CAD build for the part. Positions are in the model's coordinates, mm. A direction names the side the tool comes from. Coordinates: 2 decimals unless noted, no trailing zeros. Order: outer loops, then holes, each group sorted by start corner. A loop starts at its lowest first (then second) coordinate and runs counter-clockwise, first axis right, second up. Notation, with made-up numbers: M 38.5,-13 L 81.5,-13 A29 ccw 81.5,22 Z; hole C 87.25,46 d7. An arc over 180 degrees is marked long. Write item = value, one per line.
from build123d import *
from build123d.topology import SkipClean

# Parameters (mm, degrees)
BOSS_EXTRUDE1_DEPTH = 5.1
SKETCH2_W           = 14.45
SKETCH2_H           = 1.1
CUT_EXTRUDE1_DEPTH  = 23.625704409
SKETCH3_W           = 0.825
SKETCH3_H           = 1.1
CUT_EXTRUDE2_DEPTH  = 10
FILLET1_R           = 0.1
SKETCH4_W           = 4.1
SKETCH4_H           = 5.1
CUT_EXTRUDE3_DEPTH  = 10


with BuildPart() as part:
    # Sketch1 → Boss-Extrude1 (new body)
    with BuildSketch(Plane(origin=(0, 0, 0), x_dir=(1, 0, 0), z_dir=(0, 1, 0))):
        with BuildLine():
            Line((20.1, 4.525), (0, 4.525))
            Line((0, 4.525), (0, 2.175))
            ThreePointArc((0, 2.175), (1.537957249, 1.537957249), (2.175, 0))
            Line((2.175, 0), (20.1, 0))
            Line((20.1, 0), (20.1, 4.525))
        make_face()
        with BuildLine():
            Line((20.1, 0), (2.175, 0))
            ThreePointArc((2.175, 0), (1.537957249, -1.537957249), (0, -2.175))
            Line((0, -2.175), (0, -4.525))
            Line((0, -4.525), (20.1, -4.525))
            Line((20.1, -4.525), (20.1, 0))
        make_face()
    extrude(amount=BOSS_EXTRUDE1_DEPTH)

    # Sketch2 → Cut-Extrude1 (cut, through all)
    with BuildSketch(Plane.XY.offset(4.525)):
        with Locations((0, 4.55)):
            Rectangle(SKETCH2_W, SKETCH2_H)
    extrude(amount=-CUT_EXTRUDE1_DEPTH, mode=Mode.SUBTRACT)

    # Sketch3 → Cut-Extrude2 (cut)
    with BuildSketch(Plane.XY.offset(4.525)):
        with Locations((8.769642857, 4.55)):
            Rectangle(SKETCH3_W, SKETCH3_H)
        with Locations((10.726785714, 4.55)):
            Rectangle(SKETCH3_W, SKETCH3_H)
        with Locations((12.683928571, 4.55)):
            Rectangle(SKETCH3_W, SKETCH3_H)
        with Locations((14.641071429, 4.55)):
            Rectangle(SKETCH3_W, SKETCH3_H)
        with Locations((16.598214286, 4.55)):
            Rectangle(SKETCH3_W, SKETCH3_H)
        with Locations((18.555357143, 4.55)):
            Rectangle(SKETCH3_W, SKETCH3_H)
    extrude(amount=-CUT_EXTRUDE2_DEPTH, mode=Mode.SUBTRACT)

    # Fillet1
    fillet1_edges = [part.edges().sort_by_distance(p)[0] for p in [
        (14.228571429, 4, 0),
        (15.053571429, 4, 0),
        (17.010714286, 5.1, 0),
        (16.185714286, 5.1, 0),
        (16.185714286, 4, 0),
        (17.010714286, 4, 0),
        (18.967857143, 5.1, 0),
        (18.142857143, 5.1, 0),
        (18.142857143, 4, 0),
        (18.967857143, 4, 0),
        (20.1, 5.1, 0),
        (7.225, 4, 0),
        (7.225, 5.1, 0),
        (9.182142857, 5.1, 0),
        (8.357142857, 5.1, 0),
        (8.357142857, 4, 0),
        (9.182142857, 4, 0),
        (11.139285714, 5.1, 0),
        (10.314285714, 5.1, 0),
        (10.314285714, 4, 0),
        (11.139285714, 4, 0),
        (13.096428571, 5.1, 0),
        (12.271428571, 5.1, 0),
        (12.271428571, 4, 0),
        (13.096428571, 4, 0),
        (15.053571429, 5.1, 0),
        (14.228571429, 5.1, 0),
    ]]
    fillet(fillet1_edges, radius=FILLET1_R)

    # Mirror3: part across plane


with BuildPart() as part_1:
    with SkipClean():  # the faces are left unmerged after this step: merging them gives an invalid solid
        add(part.part)
        add(part.part.mirror(Plane(origin=(0, 5.1, 0), x_dir=(0, 0, 1), z_dir=(1, 0, 0))))

    # Sketch4 → Cut-Extrude3 (cut)
    with SkipClean():  # the faces are left unmerged after this step: merging them gives an invalid solid
        with BuildSketch(Plane.XY.offset(4.525)):
            with Locations((18.05, 2.55)):
                Rectangle(SKETCH4_W, SKETCH4_H)
            with Locations((-18.05, 2.55)):
                Rectangle(SKETCH4_W, SKETCH4_H)
        extrude(amount=-CUT_EXTRUDE3_DEPTH, mode=Mode.SUBTRACT)


solid = part_1.part
(1) Pull direction X, two halves, no side cores. Call faces 3 (the face through (15.054, 4.5, 0.1)), 4 (the face through (10, 5.1, 0)), 5 (the face through (-16, 3, 0)): +X half, -X half, draft (parallel to the pull), parting line (faces both ways), or undercut.
Evaluation:
face_3 = undercut
face_4 = draft
face_5 = -X half
(2) Wall check: line 1 (Y direction, x = -5.5, z = 1.25); line 2 (X direction, y = 3.1, z = -1.75); line 3 (X direction, y = 1.45, z = 2). Give the ranges that are in metal, low to high. Write a range as from..to.
Evaluation:
line_1 = 0..4
line_2 = -16..-1.29, 1.29..16
line_3 = -16..-0.85, 0.85..16
(3) Tool access for faces 1 (the face through (12, 5.1, 0)), 2 (the face through (8.357, 4.5, 0.1)): list every direction of +Z, -Z, +X, -X, +Y, -Y with a clear straight run to the whole face (end or side of a thin tool).
Evaluation:
face_1 = +Z, -Z, +X, -X, +Y
face_2 = +Z, -Z, +Y
(4) Slice it at B-B, the plane y = 4.7. State how many separate pieces and enclosed holes the cut face has, then the cut area to 3 significant figures.
Evaluation:
separate_pieces = 10
enclosed_holes = 0
area = 99.1 mm²
(5) Pin check, flat tip, straight feed: pin 1 Ø1.5 at (x, z) = (1, -3.5) entering from +Y. Stop position of the tip, or through.
Evaluation:
pin_1 = 4
(6) Slice it at A-A, the plane y = 3.2. Write the cut outline in (x, z) (3 decimals).
Evaluation:
outline = M -16,-4.525 L 16,-4.525 L 16,4.525 L -16,4.525 Z; hole C 0,0 d4.35
